CAD build for the part. Positions are in the model's coordinates, mm. A direction names the side the tool comes from. Give positions to 0.01 mm unless a question says otherwise; leave off trailing zeros. Order: outer loops, then holes, each group sorted by start corner. A loop starts at its lowest first (then second) coordinate and runs counter-clockwise, first axis right, second up. Notation, with made-up numbers: (74.5, 79) -> (86.5, 79) arc R23 ccw to (86.5, 87) -> close; hole circle Ø7 at (-38.75, -38). An arc over 180 degrees is marked (long way). Answer as CSV lines item,"result".
```python
from build123d import *

# Parameters (mm, degrees)
SZKIC1_R                        = 20
SZKIC1_R_2                      = 10
DODANIE_WYCI_GNI_CIE1_DEPTH     = 60
WYTNIJ_WYCI_GNI_CIE1_DEPTH      = 60
WYTNIJ_WYCI_GNI_CIE1_DEPTH_BACK = 60
SZKIC2_R                        = 7
SZKIC3_W                        = 43.38895033
SZKIC3_H                        = 20
WYTNIJ_WYCI_GNI_CIE2_DEPTH      = 35


with BuildPart() as part:
    # Szkic1 → Dodanie-wyci_gni_cie1 (new body)
    with BuildSketch(Plane.XY):
        Circle(SZKIC1_R)
        Circle(SZKIC1_R_2, mode=Mode.SUBTRACT)
    extrude(amount=DODANIE_WYCI_GNI_CIE1_DEPTH)

    # Szkic2 → Wytnij-wyci_gni_cie1 (cut, two sides: drawn at the far end of the back side and taken through both)
    with BuildSketch(Plane(origin=(0, 0, 0), x_dir=(1, 0, 0), z_dir=(0, 1, 0)).offset(-WYTNIJ_WYCI_GNI_CIE1_DEPTH_BACK)):
        with BuildLine():
            ThreePointArc((0, -60), (-14.142135624, -54.142135624), (-20, -40))
            Line((-20, -40), (-20, -60))
            Line((-20, -60), (0, -60))
        make_face()
        with BuildLine():
            Line((20, -60), (20, -40))
            ThreePointArc((20, -40), (14.142135624, -54.142135624), (0, -60))
            Line((0, -60), (20, -60))
        make_face()
        with Locations(Location((0, -40, 0), (0, 0, 90))):
            Circle(SZKIC2_R)
    extrude(amount=WYTNIJ_WYCI_GNI_CIE1_DEPTH + WYTNIJ_WYCI_GNI_CIE1_DEPTH_BACK, mode=Mode.SUBTRACT)

    # Szkic3 → Wytnij-wyci_gni_cie2 (cut)
    with BuildSketch(Plane.XY.offset(60)):
        Rectangle(SZKIC3_W, SZKIC3_H)
    extrude(amount=-WYTNIJ_WYCI_GNI_CIE2_DEPTH, mode=Mode.SUBTRACT)


solid = part.part
```
1) Pin check, flat tips, straight feed: P1, Ø3, axis at y = -14, z = 18.5, coming from the -X side; P2, Ø6, axis at x = 8.5, y = 0, coming from the +Z side; P3, Ø6, axis at x = -14.5, z = 41, coming from the +Y side. Stop position of each tip, or through.
Data:
P1,"stops at x = -15.61"
P2,"stops at z = 25"
P3,"stops at y = 16.36"
2) Pull direction Y, two halves, no side cores. Call faces 1 (the cylindrical face through (-19.98, 0.88, 22.91)), 2 (the flat face through (14, 0, 25)), 3 (the flat face through (-5, 9, 0)): pulls with the +Y half, pulls with the -Y half, needs draft (parallel to the pull), parting line crosses it, or undercut.
Data:
face 1,"parting line crosses it"
face 2,"undercut"
face 3,"needs draft"
3) Which spindle directions (+Z, -Z, +X, -X, +Y, -Y) get a long thin tool onto all of the face, cutting with end or side? Do faces 4 (the cylindrical face through (6.21, -15.08, 36.77)), 5 (the flat face through (-12, 0, 25)). Say none if no direction does.
Data:
face 4,"+Y, -Y"
face 5,"+Z, +X, -X"
4) Wall check: line 1 along X through (y, z) = (0, 11); line 2 along Z through (x, y) = (-16.5, -5.5). Give the ranges that are in metal, low to high. Write a range as [from, to].
Data:
line 1,"x = [-20, -10], [10, 20]"
line 2,"z = [0, 25]"
5) Band-saw the part on D-D, the plane z = 40. Write the cut outline in (x, y) (1 decimal), then the cut area to 3 significant figures.
Data:
outline,"(-17.3, -10) arc R20 ccw to (-7, -18.7) -> (-7, -10) -> close; (-17.3, 10) -> (-7, 10) -> (-7, 18.7) arc R20 ccw to start; (7, -18.7) arc R20 ccw to (17.3, -10) -> (7, -10) -> close; (7, 10) -> (17.3, 10) arc R20 ccw to (7, 18.7) -> close"
area,"223 mm2"
6) Band-saw the part on A-A, the plane z = 56. Write the cut outline in (x, y).
Data:
outline,"(-12, -16) arc R20 ccw to (12, -16) -> (12, -10) -> (-12, -10) -> close; (-12, 10) -> (12, 10) -> (12, 16) arc R20 ccw to (-12, 16) -> close"
7) Band-saw the part on B-B, the plane y = 0. Write the cut outline in (x, z), then the cut area to 3 significant figures.
Data:
outline,"(-20, 0) -> (-10, 0) -> (-10, 25) -> (-20, 25) -> close; (10, 0) -> (20, 0) -> (20, 25) -> (10, 25) -> close"
area,"500 mm2"
8) Band-saw the part on C-C, the plane x = -3.5. Write the cut outline in (y, z), then the cut area to 3 significant figures.
Data:
outline,"(-19.69, 0) -> (-9.37, 0) -> (-9.37, 25) -> (-10, 25) -> (-10, 33.94) -> (-19.69, 33.94) -> close; (-19.69, 46.06) -> (-10, 46.06) -> (-10, 59.69) -> (-19.69, 59.69) -> close; (9.37, 0) -> (19.69, 0) -> (19.69, 33.94) -> (10, 33.94) -> (10, 25) -> (9.37, 25) -> close; (10, 46.06) -> (19.69, 46.06) -> (19.69, 59.69) -> (10, 59.69) -> close"
area,"954 mm2"
